The listing builds one solid part. Answer for the finished solid, in the listing's coordinates (mm). A direction names the side the tool comes from. Coordinates: 2 decimals unless noted, no trailing zeros. Write each loop counter-clockwise with the first axis right and the second up, starting at its lowest first coordinate (ties: lowest second). Pieces come first, ordered by that corner, then holes. Notation, with made-up numbers: M -2.5,-25 L 8.5,-25 A26 ccw 8.5,2 Z; hole C -3.5,11.5 d1. An arc over 180 degrees is marked long. Answer as CSV lines item,"result".
```python
from build123d import *

# Parameters (mm, degrees)
BOSS_EXTRUDE1_DEPTH = 1
BOSS_EXTRUDE2_DEPTH = 2
FILLET1_R           = 1
FILLET2_R           = 2
FILLET3_R           = 3
SKETCH3_R           = 0.8
CUT_EXTRUDE1_DEPTH  = 38.344114593
CHAMFER1_SIZE       = 1


with BuildPart() as part:
    # Sketch1 → Boss-Extrude1 (new body)
    with BuildSketch(Plane.XY):
        Polygon((26.816301055, 5.1920844), (35.966301055, 5.1920844), (35.966301055, -7.1079156), (8.666301055, -7.1079156), (8.666301055, 5.1920844), (17.816301055, 5.1920844), (17.816301055, 9.5920844), (26.816301055, 9.5920844), align=None)
    extrude(amount=BOSS_EXTRUDE1_DEPTH)

    # Sketch2 → Boss-Extrude2 (add)
    with BuildSketch(Plane.XY.offset(1)):
        Polygon((34.966301055, -7.1079156), (34.966301055, 4.1920844), (25.816301055, 4.1920844), (25.816301055, 8.5920844), (18.816301055, 8.5920844), (18.816301055, 4.1920844), (9.666301055, 4.1920844), (9.666301055, -7.1079156), (8.666301055, -7.1079156), (8.666301055, 5.1920844), (17.816301055, 5.1920844), (17.816301055, 9.5920844), (26.816301055, 9.5920844), (26.816301055, 5.1920844), (35.966301055, 5.1920844), (35.966301055, -7.1079156), align=None)
    extrude(amount=BOSS_EXTRUDE2_DEPTH)

    # Fillet1
    fillet1_edges = [part.edges().sort_by_distance(p)[0] for p in [
        (9.666301055, 4.1920844, 2),
        (18.816301055, 8.5920844, 2),
        (25.816301055, 8.5920844, 2),
        (34.966301055, 4.1920844, 2),
    ]]
    fillet(fillet1_edges, radius=FILLET1_R)

    # Fillet2
    fillet2_edges = [part.edges().sort_by_distance(p)[0] for p in [
        (8.666301055, 5.1920844, 1.5),
        (17.816301055, 5.1920844, 1.5),
        (17.816301055, 9.5920844, 1.5),
        (26.816301055, 9.5920844, 1.5),
        (26.816301055, 5.1920844, 1.5),
        (35.966301055, 5.1920844, 1.5),
    ]]
    fillet(fillet2_edges, radius=FILLET2_R)

    # Fillet3
    fillet3_edges = [part.edges().sort_by_distance(p)[0] for p in [
        (18.816301055, 4.1920844, 2),
        (25.816301055, 4.1920844, 2),
    ]]
    fillet(fillet3_edges, radius=FILLET3_R)

    # Sketch3 → Cut-Extrude1 (cut, through all)
    with BuildSketch(Plane(origin=(0, 0, 0), x_dir=(-1, 0, 0), z_dir=(0, 0, -1))):
        with Locations((-32.966301055, -1.9579156)):
            Circle(SKETCH3_R)
        with Locations((-11.666301055, -1.9579156)):
            Circle(SKETCH3_R)
    extrude(amount=-CUT_EXTRUDE1_DEPTH, mode=Mode.SUBTRACT)

    # Chamfer1
    chamfer1_edges = [part.edges().sort_by_distance(p)[0] for p in [
        (13.241301055, 5.1920844, 0),
        (17.816301055, 7.3920844, 0),
        (8.666301055, -1.9579156, 0),
        (35.966301055, -1.9579156, 0),
        (22.316301055, 9.5920844, 0),
        (26.230514617, 9.006297963, 0),
        (18.402087492, 9.006297963, 0),
        (35.380514617, 4.606297963, 0),
        (9.252087492, 4.606297963, 0),
        (27.402087492, 5.777870838, 0),
        (17.230514617, 5.777870838, 0),
        (26.816301055, 7.3920844, 0),
        (31.391301055, 5.1920844, 0),
    ]]
    chamfer(chamfer1_edges, length=CHAMFER1_SIZE)


solid = part.part
```
Q1. Find section A-A (y = -3.5). Give the vertices of the cut face in (x, z), and give its area (3 significant figures).
Output:
outline,"M 8.67,1 L 9.67,0 L 34.97,0 L 35.97,1 L 35.97,3 L 34.97,3 L 34.97,1 L 9.67,1 L 9.67,3 L 8.67,3 Z"
area,"30.3 mm2"
Q2. Find section D-D (z = 0.5). Give the vertices of the cut face in (x, y).
Output:
outline,"M 9.17,-7.11 L 35.47,-7.11 L 35.47,3.19 A1.5 ccw 33.97,4.69 L 28.82,4.69 A2.5 cw 26.32,7.19 L 26.32,7.59 A1.5 ccw 24.82,9.09 L 19.82,9.09 A1.5 ccw 18.32,7.59 L 18.32,7.19 A2.5 cw 15.82,4.69 L 10.67,4.69 A1.5 ccw 9.17,3.19 Z; hole C 11.67,-1.96 d1.6; hole C 32.97,-1.96 d1.6"
Q3. The mould has two halves that part along X. Classify faces 4 (the cylindrical face through (25.516, 8.307, 2.014)), 5 (the cylindrical face through (26.718, 5.048, 2.014)), 6 (the flat face through (35.966, -2, 2)), 7 (the cylindrical face through (9.237, 4.591, 1.986)): pulls with the +X half, pulls with the -X half, needs draft (parallel to the pull), parting line crosses it, or undercut.
Output:
face 4,"undercut"
face 5,"undercut"
face 6,"pulls with the +X half"
face 7,"pulls with the -X half"
Q4. Find section B-B (z = 2.6). Give the vertices of the cut face in (x, y).
Output:
outline,"M 8.67,-7.11 L 9.67,-7.11 L 9.67,3.19 A1 cw 10.67,4.19 L 15.82,4.19 A3 ccw 18.82,7.19 L 18.82,7.59 A1 cw 19.82,8.59 L 24.82,8.59 A1 cw 25.82,7.59 L 25.82,7.19 A3 ccw 28.82,4.19 L 33.97,4.19 A1 cw 34.97,3.19 L 34.97,-7.11 L 35.97,-7.11 L 35.97,3.19 A2 ccw 33.97,5.19 L 28.82,5.19 A2 cw 26.82,7.19 L 26.82,7.59 A2 ccw 24.82,9.59 L 19.82,9.59 A2 ccw 17.82,7.59 L 17.82,7.19 A2 cw 15.82,5.19 L 10.67,5.19 A2 ccw 8.67,3.19 Z"
Q5. Find section C-C (x = 20.75). Give the vertices of the cut face in (y, z), and give its area (3 significant figures).
Output:
outline,"M -7.11,0 L 8.59,0 L 9.59,1 L 9.59,3 L 8.59,3 L 8.59,1 L -7.11,1 Z"
area,"18.2 mm2"
Q6. For faces 1 (the flat face through (22, -1, 0)), 2 (the flat face through (31, 5.192, 2)), 3 (the flat face through (34.966, -2, 2)), determine the directions among +Z, -Z, +X, -X, +Y, -Y from which every point of the face is accessible in a straight line to the end or side of a thin tool.
Output:
face 1,"-Z, +X, -X, +Y, -Y"
face 2,"+Z, -Z, +X, +Y"
face 3,"+Z, -Y"
Q7. Flat-ended cylindrical pins translate along their axes: pin 1 Ø1.6 at (x, z) = (31.5, 2) entering from +Y; pin 2 Ø0.6 at (x, z) = (23, 2) entering from -Y; pin 3 Ø1 at (x, y) = (11.67, -1.96) entering from -Z; pin 4 Ø6 at (x, y) = (18, 4.5) entering from -Z. Find the tip coordinate at first contact, or state that the pin passes through.
Output:
pin 1,"y = 5.19"
pin 2,"y = 8.59"
pin 3,"through"
pin 4,"z = 0"
Q8. Straight lines are drawn through the part: line 1 (X direction, y = -5, z = 2.45); line 2 (Z direction, x = 23.25, y = 5.25); line 3 (Y direction, x = 22.5, z = 1.95). For each, find the intervals that lie inside material, in ascending order.
Output:
line 1,"8.67 to 9.67, 34.97 to 35.97"
line 2,"0 to 1"
line 3,"8.59 to 9.59"
